Can you work these out from the model? Positions are in its coordinate system, mm. Round coordinates to 2 decimals unless told otherwise and drop trailing zeros. Loops run counter-clockwise (first coordinate to the right, second up) from the corner with the lowest first, then second, coordinate; pieces in that order, holes last.
from build123d import *

# Parameters (mm, degrees)
EXTRUDE_2_DEPTH     = 5
CUT_EXTRUDE_5_DEPTH = 173.142382928


with BuildPart() as part:
    # Эскиз4 → Бобышка-Вытянуть2 (new body)
    with BuildSketch(Plane.XY):
        Polygon((152.5, 58), (58.64, 58), (0, 38.59), (-58.64, 58), (-152.5, 58), (-162, -18.92), (-148.354716995, -23.671565122), (-86.885994913, -31.21617284), (-88.237138959, -42.15617284), (-40.597138959, -57.662313559), (40.597138959, -57.662313559), (88.237138959, -42.15617284), (86.885994913, -31.21617284), (148.354716995, -23.671565122), (162, -18.92), align=None)
        with BuildLine():
            Line((21.848195141, 15.513282482), (18.617591482, 3.873282482))
            ThreePointArc((18.617591482, 3.873282482), (0, -28.455), (-18.617591482, 3.873282482))
            Line((-18.617591482, 3.873282482), (-21.848195141, 15.513282482))
            Line((-21.848195141, 15.513282482), (-10.908195141, 11.626317085))
            ThreePointArc((-10.908195141, 11.626317085), (0, 14.595), (10.908195141, 11.626317085))
            Line((10.908195141, 11.626317085), (21.848195141, 15.513282482))
        make_face(mode=Mode.SUBTRACT)
    extrude(amount=EXTRUDE_2_DEPTH)

    # Эскиз6 → Вырез-Вытянуть5 (cut, through all)
    with BuildSketch(Plane.XY.offset(5)):
        Polygon((-144.579383614, -3.098859092), (-153.441535305, 1.018454037), (-147.02155758, 53), (-59.446003505, 53), (-18.263209753, 39.3683829), (-18.443630735, 29.370010619), (-0.197288626, 24.750877673), (18.443630735, 29.370010619), (18.263209753, 39.3683829), (59.446003505, 53), (147.02155758, 53), (153.441535305, 1.018454037), (144.579383614, -3.098859092), (146.479275056, -18.481980118), (130.103694609, -20.504445202), (127.29501371, -9.23154094), (118.988149093, -10.257479758), (118.988149093, -21.877269986), (82.262397943, -26.413081686), (83.697009804, -38.028907412), (49.312411241, -45.164872427), (46.694846048, -32.552152466), (39.076267674, -32.552152466), (38.356972556, -48.649893027), (21.981392109, -50.672358111), (-21.981392109, -50.672358111), (-38.356972556, -48.649893027), (-39.076267674, -32.552152466), (-46.694846048, -32.552152466), (-49.312411241, -45.164872427), (-83.697009804, -38.028907412), (-82.262397943, -26.413081686), (-118.988149093, -21.877269986), (-118.988149093, -10.257479758), (-127.29501371, -9.23154094), (-130.103694609, -20.504445202), (-146.479275056, -18.481980118), align=None)
    extrude(amount=-CUT_EXTRUDE_5_DEPTH, mode=Mode.SUBTRACT)


solid = part.part
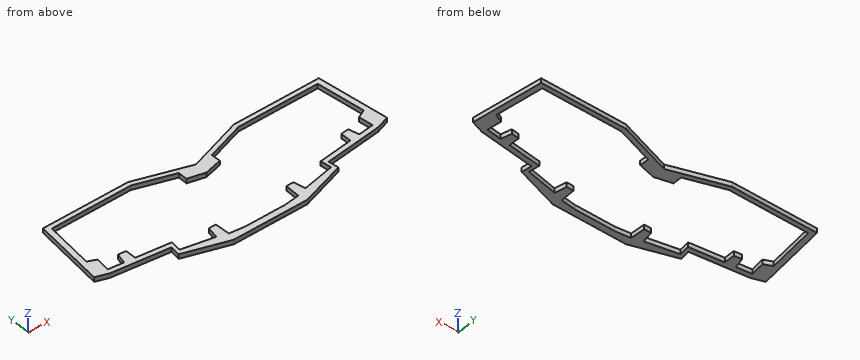
(1) If we section it at B-B, the plane y = 18: List the corners of the cut face in (x, z) for me, then the cut area to 3 significant figures.
Worked answers:
outline: (-157.44, 0) - (-151.34, 0) - (-151.34, 5) - (-157.44, 5) - close; (151.34, 0) - (157.44, 0) - (157.44, 5) - (151.34, 5) - close
area: 61.0 mm2
(2) Will these pins go through, and if not, where does the flat tip stop? P1, Ø1.5, axis at x = 119.5, z = 3, coming from the -Y side; P2, Ø2.5, axis at y = -17.5, z = 3, coming from the +X side; P3, Ø2.5, axis at x = -124.5, z = 1.5, coming from the -Y side.
Worked answers:
P1: stops at y = -27.31
P2: stops at x = 161.98
P3: stops at y = -26.75
(3) If I drill on line 1 (X direction, y = 35, z = 1.5); line 2 (Y direction, x = -13.5, z = 1.3); line 3 (Y direction, x = 4.5, z = 1.7), over which ranges is the centre line in solid material (lowest first)?
Worked answers:
line 1: x = -155.34 to -149.24, -18.34 to 18.34, 149.24 to 155.34
line 2: y = -57.66 to -50.67, 28.12 to 43.06
line 3: y = -57.66 to -50.67, 25.91 to 40.08
(4) If we section it at A-A, the plane x = 10: List the corners of the cut face in (y, z) for me.
Worked answers:
outline: (-57.66, 0) - (-50.67, 0) - (-50.67, 5) - (-57.66, 5) - close; (27.28, 0) - (41.9, 0) - (41.9, 5) - (27.28, 5) - close
